Autodesk Fusion 360 part; units mm, degrees
sketch "Sketch1" plane through (0, 0, 0) normal (0, 0, 1) x (1, 0, 0)
  line L0 (3.5, 0) -> (87.5, 0)
  line L1 (0, 3.5) -> (0, 46.5)
  line L2 (3.5, 50) -> (87.5, 50)
  line L3 (91, 46.5) -> (91, 3.5)
  line L4 (3.5, 0) -> (3.5, 50) construction
  line L5 (0, 3.5) -> (91, 3.5) construction
  circle A0 centre (3.5, 3.5) radius 1.5
  line L6 (87.5, 0) -> (87.5, 50) construction
  line L7 (0, 46.5) -> (91, 46.5) construction
  circle A1 centre (87.5, 3.5) radius 1.5
  circle A2 centre (87.5, 46.5) radius 1.5
  circle A3 centre (3.5, 46.5) radius 1.5
  arc A4 (3.5, 50) -> (0, 46.5) centre (3.5, 46.5) ccw
  arc A5 (91, 46.5) -> (87.5, 50) centre (87.5, 46.5) ccw
  arc A6 (0, 3.5) -> (3.5, 0) centre (3.5, 3.5) ccw
  arc A7 (87.5, 0) -> (91, 3.5) centre (87.5, 3.5) ccw
  circle A8 centre (3.5, 46.5) radius 3.5
  circle A9 centre (3.5, 3.5) radius 3.5
  circle A10 centre (87.5, 3.5) radius 3.5
  circle A11 centre (87.5, 46.5) radius 3.5
  line L8 (2, 51.5) -> (89, 51.5)
  line L9 (2, -1.5) -> (89, -1.5)
  line L10 (92.5, 2) -> (92.5, 48)
  line L11 (-1.5, 2) -> (-1.5, 48)
  arc A12 (92.5, 48) -> (89, 51.5) centre (89, 48) ccw
  arc A13 (2, 51.5) -> (-1.5, 48) centre (2, 48) ccw
  arc A14 (89, -1.5) -> (92.5, 2) centre (89, 2) ccw
  arc A15 (-1.5, 2) -> (2, -1.5) centre (2, 2) ccw
  line L12 (91, 7.5) -> (92.5, 7.5)
  line L13 (91, 16.5) -> (92.5, 16.5)
  line L14 (91, 44) -> (92.5, 44)
  line L15 (91, 35) -> (92.5, 35)
  line L16 (91, 12.7) -> (92.5, 12.7)
  line L17 (91, 19.7) -> (92.5, 19.7)
  line L18 (91, 5.7) -> (92.5, 5.7)
  line L19 (91, 34.8) -> (92.5, 34.8)
  line L20 (58.5, 50) -> (58.5, 51.5)
  line L21 (72.5, 50) -> (72.5, 51.5)
  line L22 (94, 20.8) -> (91, 20.8)
  point P0 (91, 0)
  point P1 (0, 50)
  point P2 (91, 50)
  dimension "d1" = 91
  dimension "d2" = 50
  dimension "d3" = 91
  dimension "d4" = 3.5
  dimension "d5" = 3.5
  dimension "d6" = 3
  dimension "d7" = 3.5
  dimension "d8" = 3.5
  dimension "d9" = 3
  dimension "d10" = 3
  dimension "d11" = 3
  dimension "d12" = 3.5
  dimension "d13" = 3.5
  dimension "d14" = 3.5
  dimension "d15" = 3.5
  dimension "d16" = 7
  dimension "d17" = 7
  dimension "d18" = 7
  dimension "d19" = 7
  dimension "d20" = 1.5
  dimension "d21" = 1.5
  dimension "d22" = 1.5
  dimension "d23" = 1.5
  dimension "d24" = 3.5
  dimension "d25" = 3.5
  dimension "d26" = 3.5
  dimension "d27" = 3.5
  dimension "d28" = 7.5
  dimension "d29" = 9
  dimension "d30" = 6
  dimension "d31" = 9
  dimension "d32" = 12.7
  dimension "d34" = 7
  dimension "d35" = 7
extrude "Extrude1" add sketch "Sketch1" along normal blind 1.5 contours L0 L1 L2 L3 A8 A9 A10 A11 | L0 L1 L2 L3 A4 A6 A7 A8 A9 A10 L8 L9 L10 L11 A13 A14 A15 L18 L20 | A6 A9 | A7 A10 | A4 A8 | L3 L10 L12 L18 | L3 L10 L12 L16 | L2 L8 L20 L21 | L3 L10 L13 L16 | L2 L3 A5 A11 L8 L10 A12 L14 L21 | L3 L10 L13 L17 | A5 A11 | L3 L10 L17 L22 | L3 L10 L19 L22 | L3 L10 L14 L15 | A0 | A1 | A2 | A3
extrude "Extrude2" add sketch "Sketch1" along normal blind 12.5 contours A6 A9 | A7 A10 | A4 A8 | A5 A11
extrude "Extrude3" add sketch "Sketch1" along normal blind 23.5 contours L0 L1 L2 L3 A4 A6 A7 A8 A9 A10 L8 L9 L10 L11 A13 A14 A15 L18 L20 | L3 L10 L12 L18 | L3 L10 L12 L16 | L2 L8 L20 L21 | L3 L10 L13 L16 | L2 L3 A5 A11 L8 L10 A12 L14 L21 | L3 L10 L13 L17 | L3 L10 L17 L22 | L3 L10 L19 L22 | L3 L10 L14 L15 | L3 L10 L15 L19
extrude "Extrude4" cut sketch "Sketch1" along normal blind 7.5 from surface at 5 contours L3 L10 L12 L18 | L3 L10 L12 L16 | L2 L8 L20 L21 | L3 L10 L13 L16 | L3 L10 L13 L17 | L3 L10 L19 L22
extrude "Extrude5" cut sketch "Sketch1" along normal blind 7.5 from surface at 14 contours L3 L10 L12 L16 | L3 L10 L13 L16
extrude "Extrude6" cut sketch "Sketch1" along normal blind 5 from surface at 14 contours L3 L10 L14 L15
The model under review builds one solid part; all positions refer to its coordinate system, in mm. A direction names the side the tool comes from. Give positions to 0.01 mm unless a question says otherwise; leave off trailing zeros. Write each loop counter-clockwise with the first axis right and the second up, starting at its lowest first coordinate (ties: lowest second). Pieces come first, ordered by that corner, then holes.
1. Add section C-C, the plane y = 26. Write out the cut boundary in (x, z).
2. Add section B-B, the plane x = 66.5. Write out the cut boundary in (y, z).
3. Draft analysis for pull direction Y (two halves, no side actions). For faces 3 (the flat face through (45, 25, 1.5)), 4 (the cylindrical face through (-0.45, -0.5, 11.59)), state which applies: +Y half, -Y half, draft (parallel to the pull), parting line (faces both ways), or undercut.
4. Add section A-A, the plane z = 8.75. Count the separate pieces of the cut face and the enclosed holes in it, plus the area to 3 significant figures.
5. Add section D-D, the plane x = 25. Write out the cut boundary in (y, z).
6. Tool access review of faces 1 (the flat face through (3, 47, 1.5)), 2 (the flat face through (45, -1.5, 12)): name each direction out of +Z, -Z, +X, -X, +Y, -Y from which nothing blocks a thin tool from reaching the whole face with its end or side.
7. Wall thickness on L1, parallel to Y at x = 12.5, z = 17.25; L2, parallel to X at y = 5.5, z = 12.75; L3, parallel to Y at x = 59, z = 10.5: over which ranges is each line inside the solid? List them lowest first.
8. For P1, Ø10, axis at x = 25.5, y = 20, coming from the -Z side; P2, Ø1.6, axis at x = 92, z = 18.5, coming from the -Y side; P3, Ø0.8, axis at y = 51, z = 10, coming from the -X side; P4, Ø3.5, axis at x = 86, y = 4, coming from the +Z side, all flat-tipped, find the tip position at first contact; note any pin that passes through.
Worked answers:
1. outline: (-1.5, 0) - (92.5, 0) - (92.5, 5) - (91, 5) - (91, 1.5) - (0, 1.5) - (0, 23.5) - (-1.5, 23.5) - close; (91, 12.5) - (92.5, 12.5) - (92.5, 23.5) - (91, 23.5) - close
2. outline: (-1.5, 0) - (51.5, 0) - (51.5, 5) - (50, 5) - (50, 1.5) - (0, 1.5) - (0, 23.5) - (-1.5, 23.5) - close; (50, 12.5) - (51.5, 12.5) - (51.5, 23.5) - (50, 23.5) - close
3. face 3: undercut
3. face 4: -Y half
4. separate pieces: 3
4. enclosed holes: 4
4. area: 495 mm2
5. outline: (-1.5, 0) - (51.5, 0) - (51.5, 23.5) - (50, 23.5) - (50, 1.5) - (0, 1.5) - (0, 23.5) - (-1.5, 23.5) - close
6. face 1: +Z
6. face 2: +Z, -Z, +X, -X, -Y
7. L1: y = -1.5 to 0, 50 to 51.5
7. L2: x = -1.5 to 0, 91 to 92.5
7. L3: y = -1.5 to 0
8. P1: stops at z = 0
8. P2: stops at y = -0.72
8. P3: stops at x = -0.34
8. P4: stops at z = 12.5
